Geometry check sheet. Reference: the model listing, model coordinates, mm. Face numbers are marked on the shaded views. Coordinates: 2 decimals unless noted, no trailing zeros. Loops run counter-clockwise (first coordinate to the right, second up) from the corner with the lowest first, then second, coordinate; pieces in that order, holes last.
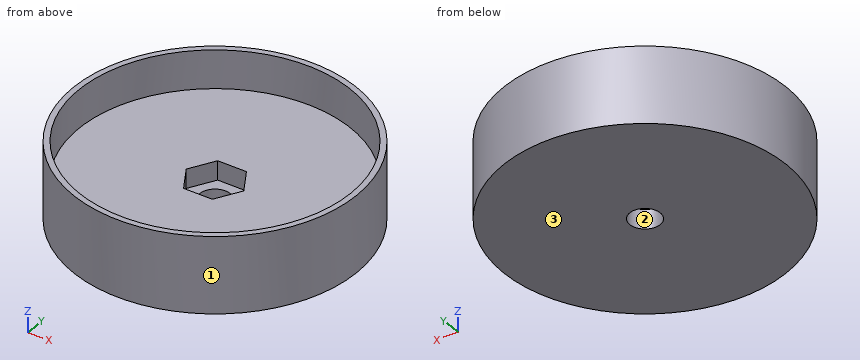
from build123d import *

# Parameters (mm, degrees)
EXTRUDE_DEPTH     = 5
CYLINDER_R        = 37
CYLINDER_DEPTH    = 20
CYLINDER001_R     = 35.5
CYLINDER001_DEPTH = 10
CYLINDER002_R     = 4
CYLINDER002_DEPTH = 5


with BuildPart() as extrude_body:
    # Polygon → Extrude (new body)
    with BuildSketch(Plane.XY):
        Polygon((7.505, 0), (3.7525, 6.499521), (-3.7525, 6.499521), (-7.505, 0), (-3.7525, -6.499521), (3.7525, -6.499521), align=None)
    extrude(amount=EXTRUDE_DEPTH)


with BuildPart() as extrude_body_1:
    # Extrude placement: moved
    add(extrude_body.part.moved(Location((0, 0, 5))))


with BuildPart() as cylinder:
    # Cylinder → Cylinder (new body)
    with BuildSketch(Plane.XY):
        Circle(CYLINDER_R)
    extrude(amount=CYLINDER_DEPTH)


with BuildPart() as cut:
    # Cut base: copy of Cylinder
    add(cylinder.part)

    # Cut: cut Extrude body
    add(extrude_body_1.part, mode=Mode.SUBTRACT)


with BuildPart() as cylinder001:
    # Cylinder001 → Cylinder001 (new body)
    with BuildSketch(Plane.XY.offset(10)):
        Circle(CYLINDER001_R)
    extrude(amount=CYLINDER001_DEPTH)


with BuildPart() as cut001:
    # Cut001 base: copy of Cylinder
    add(cylinder.part)

    # Cut001: cut Cylinder001
    add(cylinder001.part, mode=Mode.SUBTRACT)


with BuildPart() as cylinder002:
    # Cylinder002 → Cylinder002 (new body)
    with BuildSketch(Plane.XY):
        Circle(CYLINDER002_R)
    extrude(amount=CYLINDER002_DEPTH)


with BuildPart() as common:
    # Cut002 base: copy of Cylinder
    add(cylinder.part)

    # Cut002: cut Cylinder002
    add(cylinder002.part, mode=Mode.SUBTRACT)

    # Common: intersect Cut, Cut001
    add(cut.part, mode=Mode.INTERSECT)
    add(cut001.part, mode=Mode.INTERSECT)


solid = common.part
(1) Sectioned sample at A-A on z = 6. Record the cut outline in (x, y) (1 decimal).
Findings:
outline: circle Ø74 at (0, 0); hole (-7.5, 0) - (-3.8, -6.5) - (3.8, -6.5) - (7.5, 0) - (3.8, 6.5) - (-3.8, 6.5) - close
(2) Gauge pin test, flat ends, axial feed: pin 1 Ø4 at (x, z) = (0, 7.5) entering from +Y; pin 2 Ø9 at (x, y) = (0, 0) entering from +Z; pin 3 Ø3 at (x, z) = (-10.5, 3.5) entering from +Y. Record the tip position at first contact, or that the pin passes through.
Findings:
pin 1: stops at y = 37
pin 2: stops at z = 5
pin 3: stops at y = 35.89
(3) Sectioned sample at C-C on y = 29. Record the cut outline in (x, z), and give its area (3 significant figures).
Findings:
outline: (-22.98, 0) - (22.98, 0) - (22.98, 20) - (20.48, 20) - (20.48, 10) - (-20.48, 10) - (-20.48, 20) - (-22.98, 20) - close
area: 510 mm2
(4) Draft check along X on the marked faces 1, 2 and 3. Enter one of: +X half, -X half, draft (parallel to the pull), parting line (faces both ways), or undercut.
Findings:
face 1: parting line
face 2: undercut
face 3: draft
(5) Sectioned sample at D-D on x = 27.5. Record the cut outline in (y, z), and give its area (3 significant figures).
Findings:
outline: (-24.75, 0) - (24.75, 0) - (24.75, 20) - (22.45, 20) - (22.45, 10) - (-22.45, 10) - (-22.45, 20) - (-24.75, 20) - close
area: 541 mm2
(6) Scan lines: L1, parallel to Y at x = 0, z = 12; L2, parallel to Y at x = 0, z = 1.25; L3, parallel to Z at x = -12.5, y = -21. Record each from-to range of solid material in increasing order.
Findings:
L1: y = -37 to -35.5, 35.5 to 37
L2: y = -37 to -4, 4 to 37
L3: z = 0 to 10
(7) Sectioned sample at B-B on x = -2.5. Record the cut outline in (y, z), and give its area (3 significant figures).
Findings:
outline: (-36.92, 0) - (-3.12, 0) - (-3.12, 5) - (-6.5, 5) - (-6.5, 10) - (-35.41, 10) - (-35.41, 20) - (-36.92, 20) - close; (3.12, 0) - (36.92, 0) - (36.92, 20) - (35.41, 20) - (35.41, 10) - (6.5, 10) - (6.5, 5) - (3.12, 5) - close
area: 672 mm2
